Part print with two shaded views. Sizes in mm from the minimum x, y, z corner. A direction names the side the tool comes from. Round coordinates to 2 decimals unless told otherwise and drop trailing zeros. Write each loop counter-clockwise with the first axis right and the second up, starting at its lowest first coordinate (ties: lowest second). Pieces come first, ordered by that corner, then holes. Notation, with made-up numbers: (27, 10.5) - (77, 10.5) arc R29 ccw to (77, 32.5) - close; hole circle Ø8 at (89.5, 9). An arc over 180 degrees is marked (long way). Use one line per item in the form item = value. Start each with the question number.
Item 1: Pull direction Z, two halves, no side cores. Call the marked faces 3, 4, 5 and 6: +Z half, -Z half, draft (parallel to the pull), parting line (faces both ways), or undercut.
Item 2: Drill centre lines: L1, parallel to Z at x = 91, y = 1.15 (1 decimal); L2, parallel to X at y = 1.7, z = 6.5; L3, parallel to X at y = 0.9, z = 9 (1 decimal). Where is each one in solid material? Low to high.
Item 3: Band-saw the part on A-A, the plane x = 91. List the corners of the cut face in (y, z) (1 decimal), and give its area (3 significant figures).
Item 4: Band-saw the part on B-B, the plane z = 9.25. List the corners of the cut face in (x, y), and give its area (3 significant figures).
Item 5: Tool access for the marked faces 1 and 2: list every direction of +Z, -Z, +X, -X, +Y, -Y with a clear straight run to the whole face (end or side of a thin tool).
Item 6: Band-saw the part on C-C, the plane y = 1.05. List the corners of the cut face in (x, z) (1 decimal).
Item 7: Pin check, flat tip, straight feed: pin 1 (2 mm diameter, centred on x = 37, y = 5, fed in from -Z). Stop position of the tip, or through.
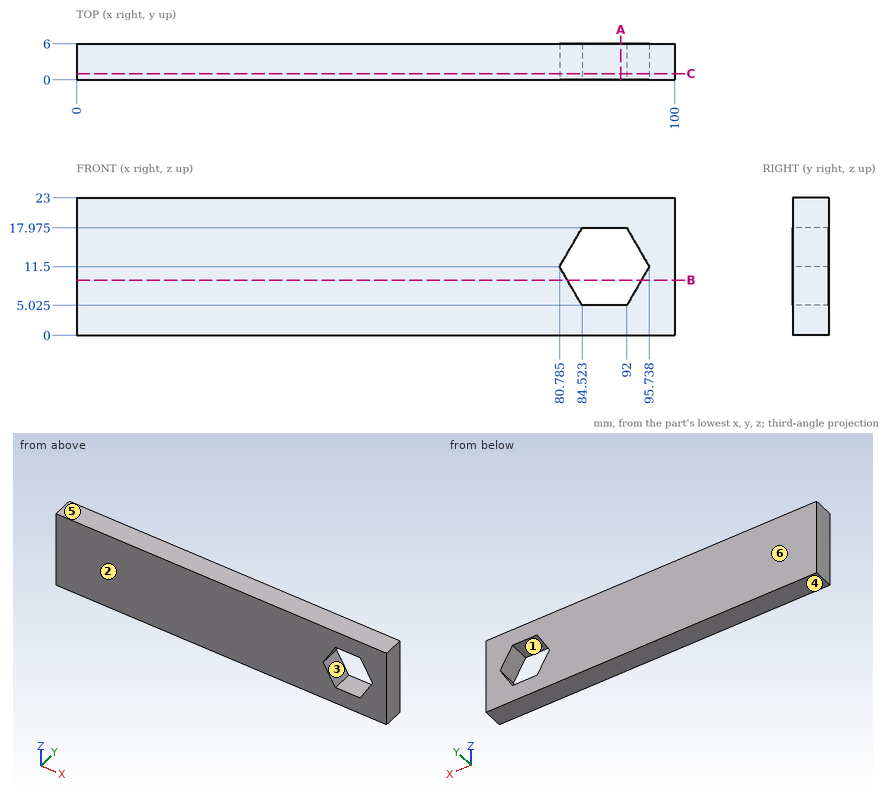
Determined:
q1.face_3 = undercut
q1.face_4 = -Z half
q1.face_5 = +Z half
q1.face_6 = draft
q2.L1 = 0 to 5, 18 to 23
q2.L2 = 0 to 83.67, 92.85 to 100
q2.L3 = 0 to 82.2, 94.3 to 100
q3.outline = (0, 0) - (6, 0) - (6, 5) - (0, 5) - close; (0, 18) - (6, 18) - (6, 23) - (0, 23) - close
q3.area = 60.3 mm²
q4.outline = (0, 0) - (82.08, 0) - (82.08, 6) - (0, 6) - close; (94.44, 0) - (100, 0) - (100, 6) - (94.44, 6) - close
q4.area = 526 mm²
q5.face_1 = +Y, -Y
q5.face_2 = +Z, -Z, +X, -X, -Y
q6.outline = (0, 0) - (100, 0) - (100, 23) - (0, 23) - close; hole (80.8, 11.5) - (84.5, 5) - (92, 5) - (95.7, 11.5) - (92, 18) - (84.5, 18) - close
q7.pin_1 = 0
